```python
from build123d import *
from build123d.topology import SkipClean

# Parameters (mm, degrees)
SZKIC1_R                               = 21
DODANIE_WYCI_GNI_CIE1_DEPTH            = 5
DODANIE_WYCI_GNI_CIE2_START            = 40
DODANIE_WYCI_GNI_CIE2_DEPTH            = 40
WYTNIJ_WYCI_GNI_CIE1_REACH             = 59.149
SZKIC4_R                               = 10
WYTNIJ_WYCI_GNI_CIE1_DIRECTION_2_DEPTH = 58.148928249
ZAOKR_GLENIE1_R                        = 10
SZKIC6_R                               = 30
DODANIE_WYCI_GNI_CIE3_DEPTH            = 5
SZKIC7_R                               = 2.5
WYTNIJ_WYCI_GNI_CIE2_DEPTH             = 5
SZYK_KO_OWY1_COUNT                     = 6


with BuildPart() as part:
    # Szkic1 → Dodanie-wyciągnięcie1 (new body)
    with BuildSketch(Plane.XY):
        Circle(SZKIC1_R)
    extrude(amount=DODANIE_WYCI_GNI_CIE1_DEPTH)

    # Szkic2 → Dodanie-wyciągnięcie2 (add)
    with SkipClean():  # the faces are left unmerged after this step: merging them gives an invalid solid
        with BuildSketch(Plane(origin=(0, 0, 0), x_dir=(-1, 0, 0), z_dir=(0, 0, -1)).offset(DODANIE_WYCI_GNI_CIE2_START)):
            with BuildLine():
                Line((-11.5, 17.571283391), (-11.5, 14))
                Line((-11.5, 14), (11.5, 14))
                Line((11.5, 14), (11.5, 17.571283391))
                ThreePointArc((11.5, 17.571283391), (0, 21), (-11.5, 17.571283391))
            make_face()
            with BuildLine():
                Line((11.5, -14), (11.5, -17.571283391))
                ThreePointArc((11.5, -17.571283391), (0, -21), (-11.5, -17.571283391))
                Line((-11.5, -17.571283391), (-11.5, -14))
                Line((-11.5, -14), (11.5, -14))
            make_face()
        extrude(amount=-DODANIE_WYCI_GNI_CIE2_DEPTH)

    # Szkic4 → Wytnij-wyciągnięcie1 (cut, up to next)
    with BuildSketch(Plane(origin=(0, -14, 0), x_dir=(1, 0, 0), z_dir=(0, 1, 0)), mode=Mode.PRIVATE) as wytnij_wyci_gni_cie1_sk1:
        with Locations(Location((0, 25, 0), (0, 0, 90))):
            Circle(SZKIC4_R)
    wytnij_wyci_gni_cie1_tool1 = extrude(wytnij_wyci_gni_cie1_sk1.sketch, amount=-WYTNIJ_WYCI_GNI_CIE1_REACH, mode=Mode.PRIVATE) & part.part
    add(wytnij_wyci_gni_cie1_tool1.solids().sort_by_distance((0, -14, -25))[0], mode=Mode.SUBTRACT)

    # Szkic4 → Wytnij-wyciągnięcie1 direction 2 (cut)
    with SkipClean():  # the faces are left unmerged after this step: merging them gives an invalid solid
        with BuildSketch(Plane(origin=(0, -14, 0), x_dir=(1, 0, 0), z_dir=(0, 1, 0))):
            with Locations(Location((0, 25, 0), (0, 0, 90))):
                Circle(SZKIC4_R)
        extrude(amount=WYTNIJ_WYCI_GNI_CIE1_DIRECTION_2_DEPTH, mode=Mode.SUBTRACT)

    # Zaokrąglenie1
    zaokr_glenie1_edges = [part.edges().sort_by_distance(p)[0] for p in [
        (0, -14, 0),
        (0, 14, 0),
    ]]
    fillet(zaokr_glenie1_edges, radius=ZAOKR_GLENIE1_R)

    # Szkic6 → Dodanie-wyciągnięcie3 (add)
    with SkipClean():  # the faces are left unmerged after this step: merging them gives an invalid solid
        with BuildSketch(Plane.XY.offset(5)):
            Circle(SZKIC6_R)
        extrude(amount=DODANIE_WYCI_GNI_CIE3_DEPTH)

    # Szkic7 → Wytnij-wyciągnięcie2 (cut)
    with SkipClean():  # the faces are left unmerged after this step: merging them gives an invalid solid
        with BuildSketch(Plane.XY.offset(10)):
            with Locations((0, 25)):
                Circle(SZKIC7_R)
        wytnij_wyci_gni_cie2 = extrude(amount=-WYTNIJ_WYCI_GNI_CIE2_DEPTH, mode=Mode.SUBTRACT)

    # Szyk kołowy1: Wytnij-wyciągnięcie2 ×6 about axis
    with SkipClean():  # the faces are left unmerged after this step: merging them gives an invalid solid
        szyk_ko_owy1_axis = Axis((0, 0, 0), (0, 0, 1))
        for i in range(1, SZYK_KO_OWY1_COUNT):
            add(wytnij_wyci_gni_cie2.rotate(szyk_ko_owy1_axis, i * 360 / SZYK_KO_OWY1_COUNT), mode=Mode.SUBTRACT)


solid = part.part
```
Check sheet for the modelled part. Datum: model origin and axes. Units: mm. A direction names the side the tool comes from. Coordinates: 2 decimals unless noted, no trailing zeros. Loops run counter-clockwise (first coordinate to the right, second up) from the corner with the lowest first, then second, coordinate; pieces in that order, holes last. Notation, with made-up numbers: M -33,5 L 20,5 A29 ccw 20,31 Z; hole C 1.25,34 d4. An arc over 180 degrees is marked long. Answer as a JSON object with one key per item and string values.
1. Sectioned sample at B-B on y = -25. Record the cut outline in (x, z).
Outcome:
{"outline": "M -16.58,5 L -2.5,5 L -2.5,10 L -16.58,10 Z; M 2.5,5 L 16.58,5 L 16.58,10 L 2.5,10 Z"}
2. Release check for a two-part mould opening along Y. For faces 6 (the cylindrical face through (-29.97, 1.32, 7.46)), 7 (the flat face through (0, -17, -40)), 8 (the cylindrical face through (-19.81, 10.81, 7.54)) record: pulls with the +Y half, pulls with the -Y half, needs draft (parallel to the pull), parting line crosses it, or undercut.
Outcome:
{"face 6": "parting line crosses it", "face 7": "needs draft", "face 8": "undercut"}
3. Sectioned sample at A-A on z = -25. Record the cut outline in (x, y), and give its area (3 significant figures).
Outcome:
{"outline": "M -11.5,-17.57 A21 ccw -10,-18.47 L -10,-14 L -11.5,-14 Z; M -11.5,14 L -10,14 L -10,18.47 A21 ccw -11.5,17.57 Z; M 10,-18.47 A21 ccw 11.5,-17.57 L 11.5,-14 L 10,-14 Z; M 10,14 L 11.5,14 L 11.5,17.57 A21 ccw 10,18.47 Z", "area": "24.2 mm²"}
4. Sectioned sample at C-C on x = 6.5. Record the cut outline in (y, z).
Outcome:
{"outline": "M -29.29,5 L -19.97,5 L -19.97,-17.4 L -14,-17.4 L -14,-10 A10 cw -4,0 L 4,0 A10 cw 14,-10 L 14,-17.4 L 19.97,-17.4 L 19.97,5 L 29.29,5 L 29.29,10 L -29.29,10 Z; M -19.97,-40 L -14,-40 L -14,-32.6 L -19.97,-32.6 Z; M 14,-40 L 19.97,-40 L 19.97,-32.6 L 14,-32.6 Z"}
5. Access from +Z, -Z, +X, -X, +Y, -Y to the whole of each face (thin tool, end or side, straight path). Record for faces 1 (the flat face through (-11.5, 15, -17)), 2 (the flat face through (0, 0, 10)), 3 (the flat face through (11.5, -15, -19)), 4 (the cylindrical face through (-0.16, 10.99, -2.85)), 5 (the flat face through (-11.3, 17.9, 5)).
Outcome:
{"face 1": "-Z, -X, +Y, -Y", "face 2": "+Z, +X, -X, +Y, -Y", "face 3": "-Z, +X, +Y, -Y", "face 4": "-Z, +X, -X", "face 5": "-Z"}
6. Depth check by flat-ended pin: P1, Ø6.5, axis at x = 21.65, y = -12.5, coming from the -Z side; P2, Ø11, axis at y = 11.5, z = -10.5, coming from the -X side; P3, Ø4, axis at y = -11, z = -17.5, coming from the -X side; P4, Ø3, axis at x = 13, z = 4, coming from the -Y side. Enter the tip coordinate at first touch or a pass-through.
Outcome:
{"P1": "z = 5", "P2": "x = -11.5", "P3": "through", "P4": "y = -27.55"}
7. Sectioned sample at D-D on y = 12.5. Record the cut outline in (x, z), and give its area (3 significant figures).
Outcome:
{"outline": "M -27.27,5 L -24.15,5 L -24.15,10 L -27.27,10 Z; M -19.15,5 L -16.87,5 L -16.87,0 L -11.5,0 L -11.5,-4.73 L 11.5,-4.73 L 11.5,0 L 16.87,0 L 16.87,5 L 19.15,5 L 19.15,10 L -19.15,10 Z; M 24.15,5 L 27.27,5 L 27.27,10 L 24.15,10 Z", "area": "500 mm²"}
8. Scan lines: L1, parallel to X at y = 12, z = 8; L2, parallel to Z at x = -8, y = 20.5; L3, parallel to X at y = -26.5, z = 7.5. Record each from-to range of solid material in increasing order. Write a range as from..to.
Outcome:
{"L1": "-27.5..-24.1, -19.2..19.2, 24.1..27.5", "L2": "5..10", "L3": "-14.06..-2, 2..14.06"}
